Design review of the part built by this model. Coordinates are the model's own, in mm. Coordinates: 2 decimals unless noted, no trailing zeros. Loops run counter-clockwise (first coordinate to the right, second up) from the corner with the lowest first, then second, coordinate; pieces in that order, holes last. Notation, with made-up numbers: (14.5, 26) -> (70.5, 26) arc R17 ccw to (70.5, 39) -> close; hole circle Ø1 at (42.5, 56). An arc over 180 degrees is marked (long way). Use a Markdown table: item, result. Add a question column.
Q1. Take a section at A-A on y = 1.6. Count the separate pieces of the cut face and the enclosed holes in it, plus the area to 3 significant figures.
Q2. For probe 1 along X at (y, z) = (2.35, -65); probe 2 along Z at (x, y) = (-8, 0.6); probe 3 along Z at (x, y) = (-6.5, 2.6), list the stretches that pass through material, from the lowest coordinate up.
Q3. Take a section at B-B on x = 3. Write out the cut boundary in (y, z), plus the area to 3 significant figures.
Q4. Take a section at D-D on z = -80. Write out the cut boundary in (x, y), plus the area to 3 significant figures.
Q5. Take a section at C-C on z = 0. Write out the cut boundary in (x, y), plus the area to 3 significant figures.
Q6. Clearance check with flat-ended pins moving along their axes: pin 1 Ø2.5 at (x, z) = (-35.52, -64.42) entering from +Y; pin 2 Ø1.5 at (x, y) = (-24, 1) entering from +Z. State where each tip first meets the part, or that it passes through.
from build123d import *

# Parameters (mm, degrees)
IZIM1_R                     = 1
IZIM1_R_2                   = 12.5
IZIM1_R_3                   = 5
IZIM1_R_4                   = 10
Y_KSEKLIK_EKSTR_ZYON1_DEPTH = 3


with BuildPart() as part:
    # Çizim1 → Yükseklik-Ekstrüzyon1 (new body)
    # profile 1 of 3: a face of its own
    with BuildSketch(Plane(origin=(0, 0, 0), x_dir=(1, 0, 0), z_dir=(0, 1, 0))):
        with BuildLine():
            ThreePointArc((0, -12.5), (-11.543595981, -4.795351063), (-8.856895242, 8.820737309))
            ThreePointArc((-8.856895242, 8.820737309), (-25.386606646, 21.485478314), (-29.697678368, 41.85805018))
            ThreePointArc((-29.697678368, 41.85805018), (-2.160717, 110.170160276), (56.238508843, 155.051771745))
            ThreePointArc((56.238508843, 155.051771745), (43.192574473, 160.511038766), (48.651841494, 173.556973137))
            ThreePointArc((48.651841494, 173.556973137), (-18.46803273, 121.763907855), (-49.702354676, 42.947562724))
            ThreePointArc((-49.702354676, 42.947562724), (-37.231560108, 4.126193926), (0, -12.5))
        make_face()
        with Locations(Location((-39.761883741, 41.85805018, 0), (0, 0, 270))):
            Circle(IZIM1_R, mode=Mode.SUBTRACT)
        with Locations(Location((-35.520748055, 64.423751915, 0), (0, 0, 270))):
            Circle(IZIM1_R, mode=Mode.SUBTRACT)
        with Locations(Location((-27.885254768, 86.077790082, 0), (0, 0, 270))):
            Circle(IZIM1_R, mode=Mode.SUBTRACT)
        with Locations(Location((-17.034311334, 106.31278831, 0), (0, 0, 270))):
            Circle(IZIM1_R, mode=Mode.SUBTRACT)
        with Locations(Location((-3.222166513, 124.654619792, 0), (0, 0, 270))):
            Circle(IZIM1_R, mode=Mode.SUBTRACT)
        with Locations(Location((13.227546947, 140.673516564, 0), (0, 0, 270))):
            Circle(IZIM1_R, mode=Mode.SUBTRACT)
        with Locations(Location((31.929395352, 153.994139408, 0), (0, 0, 270))):
            Circle(IZIM1_R, mode=Mode.SUBTRACT)
    # profile 2 of 3: a face of its own
    with BuildSketch(Plane(origin=(0, 0, 0), x_dir=(1, 0, 0), z_dir=(0, 1, 0))):
        Circle(IZIM1_R_2)
        with Locations(Location((0, 0, 0), (0, 0, 270))):
            Circle(IZIM1_R_3, mode=Mode.SUBTRACT)
    # profile 3 of 3: a face of its own
    with BuildSketch(Plane(origin=(0, 0, 0), x_dir=(1, 0, 0), z_dir=(0, 1, 0))):
        with Locations((52.445175169, 164.304372441)):
            Circle(IZIM1_R_4)
        with Locations(Location((52.445175169, 164.304372441, 0), (0, 0, 270))):
            Circle(IZIM1_R, mode=Mode.SUBTRACT)
    extrude(amount=Y_KSEKLIK_EKSTR_ZYON1_DEPTH)


solid = part.part
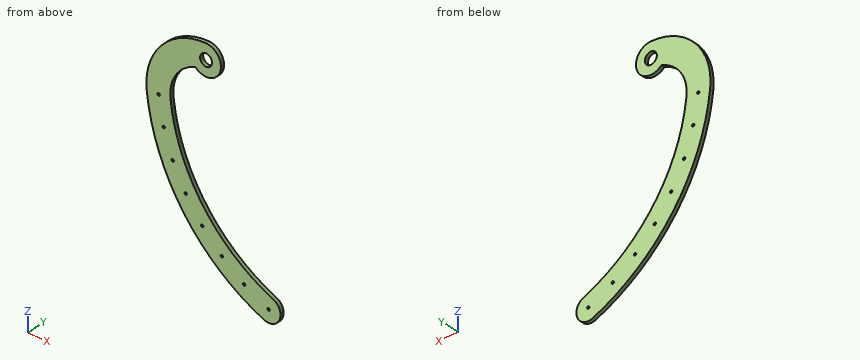
Answer list:
| question | item | result |
|---|---|---|
| 1 | separate pieces | 1 |
| 1 | enclosed holes | 9 |
| 1 | area | 4,890 mm² |
| 2 | probe 1 | -45.71 to -36.34, -34.7 to -24.97 |
| 2 | probe 2 | -134.28 to -101.87, -9.6 to 11.86 |
| 2 | probe 3 | -135.88 to -104.13, -10.68 to 12.08 |
| 3 | outline | (0, -145.06) -> (3, -145.06) -> (3, -116.57) -> (0, -116.57) -> close; (0, -12.13) -> (3, -12.13) -> (3, -4) -> (0, -4) -> close; (0, 4) -> (3, 4) -> (3, 12.13) -> (0, 12.13) -> close |
| 3 | area | 134 mm² |
| 4 | outline | (-41.09, 0) -> (-19.62, 0) -> (-19.62, 3) -> (-41.09, 3) -> close |
| 4 | area | 64.4 mm² |
| 5 | outline | (-33.07, 0) -> (-5, 0) -> (-5, 3) -> (-33.07, 3) -> close; (5, 0) -> (12.5, 0) -> (12.5, 3) -> (5, 3) -> close |
| 5 | area | 107 mm² |
| 6 | pin 1 | y = 3 |
| 6 | pin 2 | z = 6.77 |
